```python
from build123d import *

# Parameters (mm, degrees)
SKETCH_R     = 1.45
SKETCH_R_2   = 15
PAD_DEPTH    = 3
PAD001_DEPTH = 12


with BuildPart() as part:
    # Sketch → Pad (new body)
    with BuildSketch(Plane.XY):
        with BuildLine():
            Line((-12, 16.5), (12, 16.5))
            ThreePointArc((16.5, 12), (15.181981, 15.181981), (12, 16.5))
            Line((16.5, 12), (16.5, -12))
            Line((16.5, -38.5), (16.5, -12))
            Line((41.5, -38.5), (16.5, -38.5))
            Line((41.5, -41.5), (41.5, -38.5))
            Line((-26.5, -41.5), (41.5, -41.5))
            Line((-16.5, -12), (-26.5, -41.5))
            Line((-16.5, -12), (-16.5, 12))
            ThreePointArc((-12, 16.5), (-15.181981, 15.181981), (-16.5, 12))
        make_face()
        with Locations((-12, 12)):
            Circle(SKETCH_R, mode=Mode.SUBTRACT)
        with Locations((12, 12)):
            Circle(SKETCH_R, mode=Mode.SUBTRACT)
        with Locations((-12, -12)):
            Circle(SKETCH_R, mode=Mode.SUBTRACT)
        with Locations((12, -12)):
            Circle(SKETCH_R, mode=Mode.SUBTRACT)
        Circle(SKETCH_R_2, mode=Mode.SUBTRACT)
    extrude(amount=PAD_DEPTH)

    # Sketch001 (on DatumPlane) → Pad001 (join)
    with BuildSketch(Plane.XY.offset(3)):
        Polygon((41.5, -38.5), (-25.483051, -38.5), (-26.5, -41.5), (41.5, -41.5), align=None)
    extrude(amount=PAD001_DEPTH)


solid = part.part
```
Here's how the part is built. I have some questions about the finished solid (model axes, mm). A direction names the side the tool comes from. Give positions to 0.01 mm unless a question says otherwise; leave off trailing zeros. Write each loop counter-clockwise with the first axis right and the second up, starting at its lowest first coordinate (ties: lowest second). Pieces come first, ordered by that corner, then holes. Notation, with made-up numbers: M -1,42.5 L 22,42.5 A19 cw 22,62.5 Z; hole C 83.25,2 d1. An arc over 180 degrees is marked long. Put each result on its own line as item: value. Start each with the question number.
Item 1: Thinking about a two-plate mould opening in X: for faces 4 (the flat face through (0, -19, 0)), 5 (the cylindrical face through (15.217, 15.147, 1.479)), 6 (the cylindrical face through (-14.985, 0.66, 1.479)), which applies, +X half, -X half, draft (parallel to the pull), parting line (faces both ways), or undercut?
Item 2: If we section it at D-D, the plane z = 13.25: Write out the boundary of the cut face in (x, y), then the cut area to 3 significant figures.
Item 3: If we section it at A-A, the plane y = 0: Write out the boundary of the cut face in (x, z).
Item 4: On a 3-axis mill with a long thin cutter (end or side, diameter ignored), from which of +Z, -Z, +X, -X, +Y, -Y can I reach the whole of each face in a straight line? I mean faces 1 (the flat face through (-16.5, 0, 1)), 2 (the flat face through (16.5, -14, 1)), 3 (the flat face through (0, -17, 3)). Say none if no direction works.
Item 5: Will these pins go through, and if not, where does the flat tip stop? pin 1 (2.5 mm diameter, centred on x = -12, y = 12, fed in from +Z); pin 2 (6 mm diameter, centred on x = 29, z = 13, fed in from +Y); pin 3 (12 mm diameter, centred on x = -17, y = -12.5, fed in from +Z); pin 4 (1.5 mm diameter, centred on y = -17.5, z = 1, fed in from +X).
Item 6: If we section it at B-B, the plane z = 1.75: Write out the boundary of the cut face in (x, y), then the cut area to 3 significant figures.
Item 7: I need wall thicknesses on L1, parallel to Y at x = 12, z = 1.3; L2, parallel to Y at x = 0, z = 0.9; L3, parallel to Y at x = 30.5, z = 7.5. Which ranges of each line are inside material? Lowest first, please. Write a range as from..to.
Item 8: If we section it at C-C, the plane x = 34: Write out the boundary of the cut face in (y, z).
Values:
1. face 4: draft
1. face 5: +X half
1. face 6: undercut
2. outline: M -26.5,-41.5 L 41.5,-41.5 L 41.5,-38.5 L -25.48,-38.5 Z
2. area: 202 mm²
3. outline: M -16.5,0 L -15,0 L -15,3 L -16.5,3 Z; M 15,0 L 16.5,0 L 16.5,3 L 15,3 Z
4. face 1: +Z, -Z, -X, +Y
4. face 2: +Z, -Z, +X, +Y
4. face 3: +Z, +X, -X, +Y
5. pin 1: through
5. pin 2: y = -38.5
5. pin 3: z = 3
5. pin 4: x = 16.5
6. outline: M -26.5,-41.5 L 41.5,-41.5 L 41.5,-38.5 L 16.5,-38.5 L 16.5,12 A4.5 ccw 12,16.5 L -12,16.5 A4.5 ccw -16.5,12 L -16.5,-12 Z; hole C 0,0 d30; hole C -12,-12 d2.9; hole C -12,12 d2.9; hole C 12,-12 d2.9; hole C 12,12 d2.9
6. area: 1,390 mm²
7. L1: -41.5..-13.45, -10.55..-9, 9..10.55, 13.45..16.5
7. L2: -41.5..-15, 15..16.5
7. L3: -41.5..-38.5
8. outline: M -41.5,0 L -38.5,0 L -38.5,15 L -41.5,15 Z
